```python
from build123d import *

# Parameters (mm, degrees)
SKETCH1_W               = 12.7
SKETCH1_H               = 25.4
SKETCH1_W_2             = 6.35
SKETCH1_H_2             = 19.05
BOSS_EXTRUDE1_DEPTH     = 558.8
CUT_EXTRUDE1_DEPTH      = 560.088561858
CUT_EXTRUDE1_DEPTH_BACK = 560.088561858
SKETCH2_R               = 3.3528
CUT_EXTRUDE2_REACH      = 561.089
SKETCH3_R               = 3.937


with BuildPart() as part:
    # Sketch1 → Boss-Extrude1 (new body)
    with BuildSketch(Plane(origin=(0, 0, 0), x_dir=(0, 0, -1), z_dir=(1, 0, 0))):
        Rectangle(SKETCH1_W, SKETCH1_H)
        Rectangle(SKETCH1_W_2, SKETCH1_H_2, mode=Mode.SUBTRACT)
    extrude(amount=BOSS_EXTRUDE1_DEPTH)

    # Sketch2 → Cut-Extrude1 (cut, two sides: drawn at the far end of the back side and taken through both)
    with BuildSketch(Plane.XY.offset(6.35).offset(-CUT_EXTRUDE1_DEPTH_BACK)):
        with Locations((546.1, 0)):
            Circle(SKETCH2_R)
        with Locations(Location((12.7, 0, 0), (0, 0, 270))):
            Circle(SKETCH2_R)
    extrude(amount=CUT_EXTRUDE1_DEPTH + CUT_EXTRUDE1_DEPTH_BACK, mode=Mode.SUBTRACT)

    # Sketch3 → Cut-Extrude2 (cut, up to next)
    with BuildSketch(Plane.XY.offset(6.35), mode=Mode.PRIVATE) as cut_extrude2_sk1:
        with Locations((546.1, 0)):
            Circle(SKETCH3_R)
    cut_extrude2_tool1 = extrude(cut_extrude2_sk1.sketch, amount=-CUT_EXTRUDE2_REACH, mode=Mode.PRIVATE) & part.part
    # Sketch3 → Cut-Extrude2 (cut, up to next)
    with BuildSketch(Plane.XY.offset(6.35), mode=Mode.PRIVATE) as cut_extrude2_sk2:
        with Locations((12.7, 0)):
            Circle(SKETCH3_R)
    cut_extrude2_tool2 = extrude(cut_extrude2_sk2.sketch, amount=-CUT_EXTRUDE2_REACH, mode=Mode.PRIVATE) & part.part
    add(cut_extrude2_tool1.solids().sort_by_distance((546.1, 0, 6.35))[0], mode=Mode.SUBTRACT)
    add(cut_extrude2_tool2.solids().sort_by_distance((12.7, 0, 6.35))[0], mode=Mode.SUBTRACT)


solid = part.part
```
Check sheet for the modelled part. Datum: model origin and axes. Units: mm. A direction names the side the tool comes from. Give positions to 0.01 mm unless a question says otherwise; leave off trailing zeros. Order: outer loops, then holes, each group sorted by start corner. A loop starts at its lowest first (then second) coordinate and runs counter-clockwise, first axis right, second up. Notation, with made-up numbers: M 36.25,56.25 L 60.25,56.25 A11 cw 60.25,70.25 Z; hole C -16,-13 d8. An arc over 180 degrees is marked long. Answer in a Markdown table with one row per item. Add a question column.
Q1. Sectioned sample at A-A, the plane z = -0.25. Record the boundary of the cut face in (x, y) (3 decimals).
Q2. Sectioned sample at B-B, the plane x = 479.5. Record the boundary of the cut face in (y, z) (3 decimals).
Q3. Release check for a two-part mould opening along Z. For faces 3 (the flat face through (275, 0, 3.175)), 4 (the flat face through (275, 0, -6.35)), 5 (the flat face through (275, 0, 6.35)), 6 (the flat face through (0, 0, -4)) record: released by +Z, released by -Z, zero draft, split by the parting line, or undercut.
Q4. Thickness scan on L1, parallel to X at y = 0, z = -4.8; L2, parallel to Y at x = 476.5, z = -2.5 (3 decimals); L3, parallel to X at y = -0.5, z = -3.75. Record the ranges inside material, lowest first.
Q5. Access from +Z, -Z, +X, -X, +Y, -Y to the whole of each face (thin tool, end or side, straight path). Record for faces 1 (the flat face through (558.8, 0, -4)), 2 (the flat face through (275, 0, -3.175)).
Verdict:
| question | item | result |
|---|---|---|
| 1 | outline | M 0,-12.7 L 558.8,-12.7 L 558.8,-9.525 L 0,-9.525 Z; M 0,9.525 L 558.8,9.525 L 558.8,12.7 L 0,12.7 Z |
| 2 | outline | M -12.7,-6.35 L 12.7,-6.35 L 12.7,6.35 L -12.7,6.35 Z; hole M -9.525,-3.175 L 9.525,-3.175 L 9.525,3.175 L -9.525,3.175 Z |
| 3 | face 3 | undercut |
| 3 | face 4 | released by -Z |
| 3 | face 5 | released by +Z |
| 3 | face 6 | zero draft |
| 4 | L1 | 0 to 9.35, 16.05 to 542.75, 549.45 to 558.8 |
| 4 | L2 | -12.7 to -9.525, 9.525 to 12.7 |
| 4 | L3 | 0 to 9.38, 16.02 to 542.78, 549.42 to 558.8 |
| 5 | face 1 | +Z, -Z, +X, +Y, -Y |
| 5 | face 2 | +X, -X |
